Source: CAD feature listing. Evaluate the final solid. Frame: model axes, mm. Face numbers are marked on the shaded views. A direction names the side the tool comes from. Round coordinates to 2 decimals unless told otherwise and drop trailing zeros. Order: outer loops, then holes, each group sorted by start corner. A loop starts at its lowest first (then second) coordinate and runs counter-clockwise, first axis right, second up. Notation, with made-up numbers: (33, 85) -> (80, 85) arc R34 cw to (80, 117) -> close; hole circle Ø4 at (-17, 29). An arc over 180 degrees is marked (long way). One line per item, written item: value. Start each with the question number.
1) Ray query, L1, parallel to Y at x = 22.5, z = 63.5; L2, parallel to X at y = 13, z = 46; L3, parallel to Z at x = 6, y = 25. Return the intervals inside material, ascending.
2) Section C-C (x = 22.5). Return the cut outline in (y, z), and give its area (3 significant figures).
3) Reachability of the marked faces 4, 5 and 6 from +Z, -Z, +X, -X, +Y, -Y: full face, straight path, thin tool, end or side. Return the list, or none.
4) Pin query (flat end, axial travel): P1, Ø23, axis at y = 25, z = 40, coming from the +X side; P2, Ø5, axis at x = 54, y = 15.5, coming from the +Z side; P3, Ø1.5, axis at x = 24.5, y = 20, coming from the +Z side. Return the tip coordinate at first contact, or that it passes through.
5) Section A-A (z = 40). Return the cut outline in (x, y), and give its area (3 significant figures).
6) Section B-B (y = 25). Return the cut outline in (x, z).
7) Mould query, pull axis X, two halves, no side actions, for the marked faces 1, 2 and 3. Classes: pulls with the +X half, pulls with the -X half, needs draft (parallel to the pull), parting line crosses it, or undercut.
8) Section D-D (z = 16.5). Return the cut outline in (x, y).
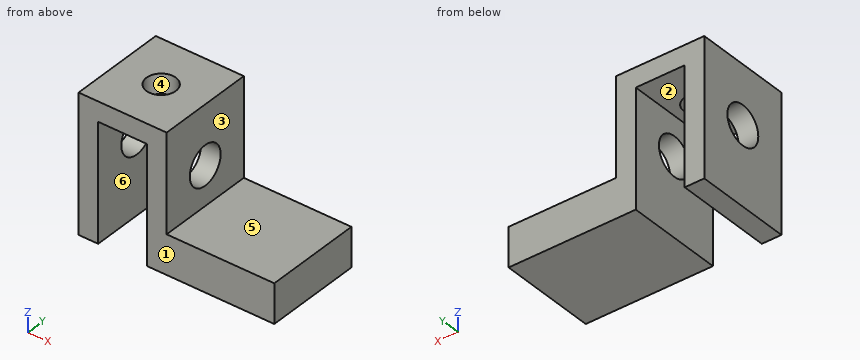
```python
from build123d import *

# Parameters (mm, degrees)
F0_W      = 100
F0_H      = 50
F1_DEPTH  = 20
F2_W      = 45
F2_H      = 50
F3_DEPTH  = 50
F4_W      = 25
F4_H      = 60
F5_DEPTH  = 50.001
F6_R      = 10
F7_DEPTH  = 100.001
F8_R      = 7.5
F10_DEPTH = 70.001


# Not quite as in the source:
# - a feature of the source that left no trace in its solid (it failed there, or was rolled back) is left out


with BuildPart() as f1:
    # F0 (on Top) → F1 (new body)
    with BuildSketch(Plane.XY):
        with Locations((50, 25)):
            Rectangle(F0_W, F0_H)
    extrude(amount=F1_DEPTH)

    # F2 (on face) → F3 (join)
    with BuildSketch(Plane.XY.offset(20)):
        with Locations((22.5, 25)):
            Rectangle(F2_W, F2_H)
    extrude(amount=F3_DEPTH)

    # F4 (on face) → F5 (cut, through all)
    with BuildSketch(Plane.XZ):
        with Locations((22.5, 30)):
            Rectangle(F4_W, F4_H)
    extrude(amount=-F5_DEPTH, mode=Mode.SUBTRACT)

    # F6 (on face) → F7 (cut, through all)
    with BuildSketch(Plane(origin=(0, 0, 0), x_dir=(0, -1, 0), z_dir=(-1, 0, 0))):
        with Locations((-25, 40)):
            Circle(F6_R)
    extrude(amount=-F7_DEPTH, mode=Mode.SUBTRACT)

    # F8 (on face) → F10 (cut, through all)
    with BuildSketch(Plane.XY.offset(70)):
        with Locations((22.5, 25)):
            Circle(F8_R)
    extrude(amount=-F10_DEPTH, mode=Mode.SUBTRACT)


solid = f1.part
```
Findings:
1. L1: 0 to 17.5, 32.5 to 50
1. L2: 0 to 10, 35 to 45
1. L3: 0 to 30, 50 to 70
2. outline: (0, 60) -> (17.5, 60) -> (17.5, 70) -> (0, 70) -> close; (32.5, 60) -> (50, 60) -> (50, 70) -> (32.5, 70) -> close
2. area: 350 mm2
3. face 4: +Z, -Z
3. face 5: +Z, +X, +Y, -Y
3. face 6: -Z, +Y, -Y
4. P1: x = 45
4. P2: z = 20
4. P3: through
5. outline: (0, 0) -> (10, 0) -> (10, 15) -> (0, 15) -> close; (0, 35) -> (10, 35) -> (10, 50) -> (0, 50) -> close; (35, 0) -> (45, 0) -> (45, 15) -> (35, 15) -> close; (35, 35) -> (45, 35) -> (45, 50) -> (35, 50) -> close
5. area: 600 mm2
6. outline: (0, 0) -> (10, 0) -> (10, 30) -> (0, 30) -> close; (0, 50) -> (10, 50) -> (10, 60) -> (15, 60) -> (15, 70) -> (0, 70) -> close; (30, 60) -> (35, 60) -> (35, 50) -> (45, 50) -> (45, 70) -> (30, 70) -> close; (35, 0) -> (100, 0) -> (100, 20) -> (45, 20) -> (45, 30) -> (35, 30) -> close
7. face 1: needs draft
7. face 2: undercut
7. face 3: pulls with the +X half
8. outline: (0, 0) -> (10, 0) -> (10, 50) -> (0, 50) -> close; (35, 0) -> (100, 0) -> (100, 50) -> (35, 50) -> close
